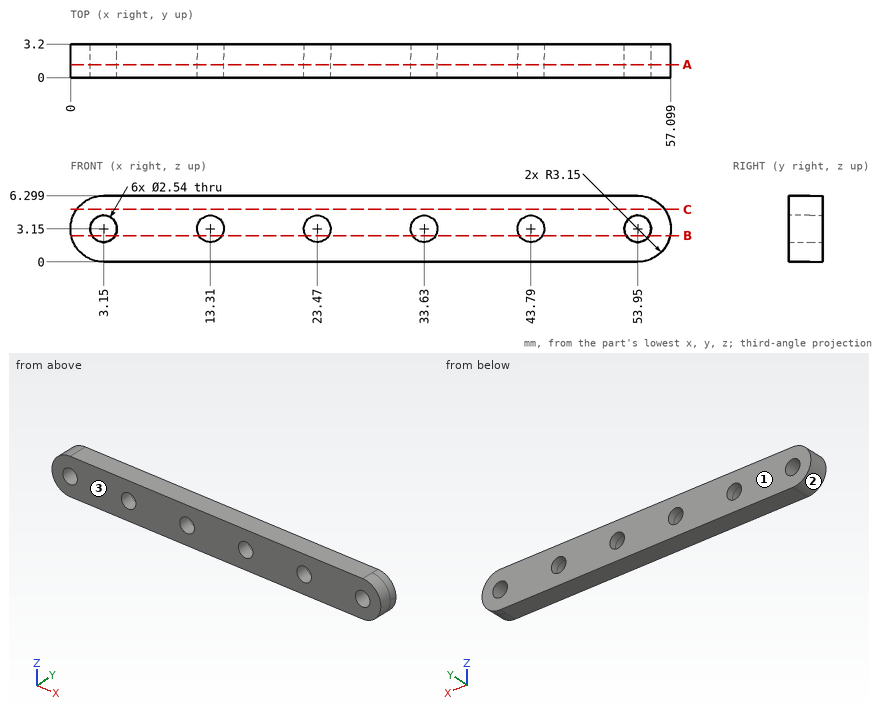
Part print with two shaded views. Sizes in mm from the minimum x, y, z corner. Round coordinates to 2 decimals unless told otherwise and drop trailing zeros. Loops run counter-clockwise (first coordinate to the right, second up) from the corner with the lowest first, then second, coordinate; pieces in that order, holes last. Notation, with made-up numbers: M 52,77 L 102,77 A11 ccw 102,83 Z; hole C -1.5,68.5 d1. An arc over 180 degrees is marked long. Return JSON: item names as keys, results as strings. Group by question number.
(1) Saw through at A-A, the plane y = 1.25. List the corners of the cut face in (x, z).
(2) Mould opens along Y. For the marked faces 1, 2 and 3 say: +Y half, -Y half, draft (parallel to the pull), parting line (faces both ways), or undercut.
(3) Saw through at C-C, the plane z = 5. List the corners of the cut face in (x, y), and give its area (3 significant figures).
(4) Wall check: probe 1 along Z at (x, y) = (44, 2.15); probe 2 along Z at (x, y) = (22.5, 1.65); probe 3 along X at (y, z) = (2.1, 5.5) (1 decimal). Give the ranges that are in metal, low to high. Write a range as [from, to].
(5) Saw through at B-B, the plane z = 2.5. List the corners of the cut face in (x, y).
Answer list:
{
 "1": {"outline": "M 3.15,0 L 53.95,0 A3.15 ccw 53.95,6.3 L 3.15,6.3 A3.15 ccw Z; hole C 3.15,3.15 d2.54; hole C 13.31,3.15 d2.54; hole C 23.47,3.15 d2.54; hole C 33.63,3.15 d2.54; hole C 43.79,3.15 d2.54; hole C 53.95,3.15 d2.54"},
 "2": {"face 1": "+Y half", "face 2": "draft", "face 3": "-Y half"},
 "3": {"outline": "M 0.6,0 L 56.5,0 L 56.5,3.2 L 0.6,3.2 Z", "area": "179 mm2"},
 "4": {"probe 1": "[0, 1.9], [4.4, 6.3]", "probe 2": "[0, 2.33], [3.97, 6.3]", "probe 3": "[1.1, 56]"},
 "5": {"outline": "M 0.07,0 L 2.06,0 L 2.06,3.2 L 0.07,3.2 Z; M 4.24,0 L 12.22,0 L 12.22,3.2 L 4.24,3.2 Z; M 14.4,0 L 22.38,0 L 22.38,3.2 L 14.4,3.2 Z; M 24.56,0 L 32.54,0 L 32.54,3.2 L 24.56,3.2 Z; M 34.72,0 L 42.7,0 L 42.7,3.2 L 34.72,3.2 Z; M 44.88,0 L 52.86,0 L 52.86,3.2 L 44.88,3.2 Z; M 55.04,0 L 57.03,0 L 57.03,3.2 L 55.04,3.2 Z"}
}
